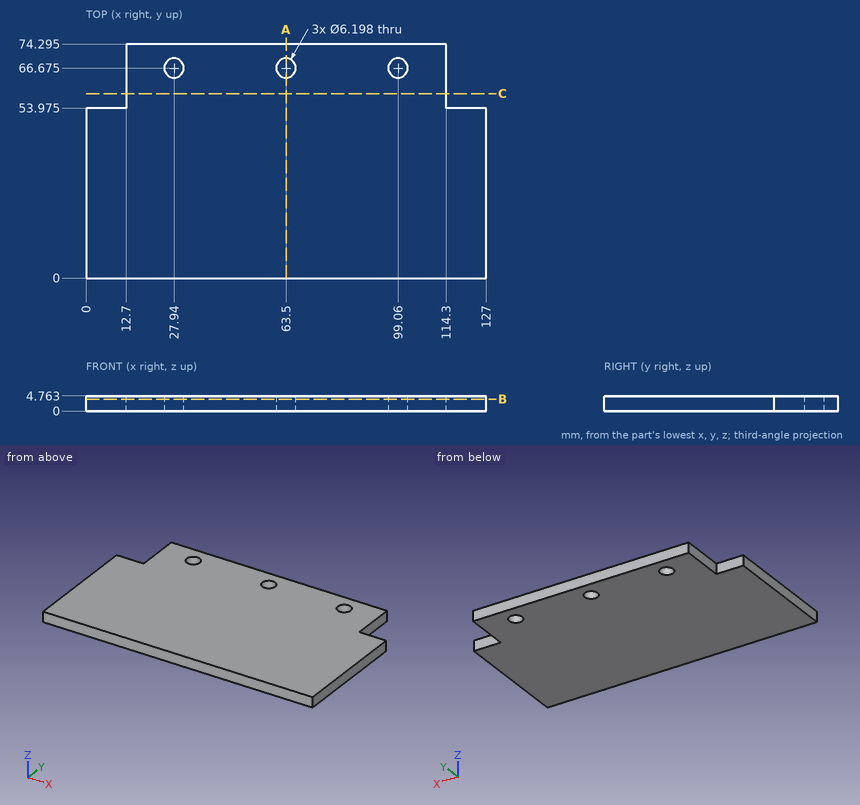
Design review of the part shown in the three views and the two pictorial views. Dimensions are in mm from the part's minimum x, y and z. Round coordinates to 2 decimals unless told otherwise and drop trailing zeros. Write each loop counter-clockwise with the first axis right and the second up, starting at its lowest first coordinate (ties: lowest second). Pieces come first, ordered by that corner, then holes.
Item 1: For probe 1 along Y at (x, z) = (27.94, 3.1) (1 decimal); probe 2 along Y at (x, z) = (118.5, 4.1) (1 decimal); probe 3 along Y at (x, z) = (27, 2.25) (1 decimal), list the stretches that pass through material, from the lowest coordinate up.
Item 2: We need section B-B on z = 3.8. Write out the cut boundary in (x, y) (1 decimal).
Item 3: We need section C-C on y = 58.5. Write out the cut boundary in (x, z).
Item 4: Clearance check with flat-ended pins moving along their axes: pin 1 Ø2.5 at (y, z) = (60, 1.5) entering from +X; pin 2 Ø5 at (x, y) = (63.5, 66.675) entering from +Z; pin 3 Ø2.5 at (y, z) = (64, 1.5) entering from -X. State where each tip first meets the part, or that it passes through.
Item 5: We need section A-A on x = 63.5. Write out the cut boundary in (y, z) (1 decimal).
Returned:
1. probe 1: y = 0 to 63.6, 69.8 to 74.3
1. probe 2: y = 0 to 54
1. probe 3: y = 0 to 63.7, 69.6 to 74.3
2. outline: (0, 0) - (127, 0) - (127, 54) - (114.3, 54) - (114.3, 74.3) - (12.7, 74.3) - (12.7, 54) - (0, 54) - close; hole circle Ø6.2 at (27.9, 66.7); hole circle Ø6.2 at (63.5, 66.7); hole circle Ø6.2 at (99.1, 66.7)
3. outline: (12.7, 0) - (114.3, 0) - (114.3, 4.76) - (12.7, 4.76) - close
4. pin 1: stops at x = 114.3
4. pin 2: passes through
4. pin 3: stops at x = 12.7
5. outline: (0, 0) - (63.6, 0) - (63.6, 4.8) - (0, 4.8) - close; (69.8, 0) - (74.3, 0) - (74.3, 4.8) - (69.8, 4.8) - close
